from build123d import *

# Parameters (mm, degrees)
SKETCH1_W           = 25.4
SKETCH1_H           = 25.4
SKETCH1_W_2         = 20.32
SKETCH1_H_2         = 20.32
BOSS_EXTRUDE1_DEPTH = 139.7
SKETCH2_R           = 2.032
CUT_EXTRUDE1_DEPTH  = 143.557146436
SKETCH3_R           = 2.032
CUT_EXTRUDE2_DEPTH  = 143.557146436


with BuildPart() as part:
    # Sketch1 → Boss-Extrude1 (new body)
    with BuildSketch(Plane(origin=(0, 0, 0), x_dir=(0, 0, -1), z_dir=(1, 0, 0))):
        Rectangle(SKETCH1_W, SKETCH1_H)
        Rectangle(SKETCH1_W_2, SKETCH1_H_2, mode=Mode.SUBTRACT)
    extrude(amount=BOSS_EXTRUDE1_DEPTH)

    # Sketch2 → Cut-Extrude1 (cut, through all)
    with BuildSketch(Plane(origin=(0, 12.7, 0), x_dir=(1, 0, 0), z_dir=(0, 1, 0))):
        Circle(SKETCH2_R)
        with Locations(Location((12.7, 0, 0), (0, 0, 270))):
            Circle(SKETCH2_R)
        with Locations(Location((25.4, 0, 0), (0, 0, 270))):
            Circle(SKETCH2_R)
        with Locations(Location((38.1, 0, 0), (0, 0, 270))):
            Circle(SKETCH2_R)
        with Locations(Location((50.8, 0, 0), (0, 0, 270))):
            Circle(SKETCH2_R)
        with Locations(Location((63.5, 0, 0), (0, 0, 270))):
            Circle(SKETCH2_R)
        with Locations(Location((76.2, 0, 0), (0, 0, 270))):
            Circle(SKETCH2_R)
        with Locations(Location((88.9, 0, 0), (0, 0, 270))):
            Circle(SKETCH2_R)
        with Locations(Location((101.6, 0, 0), (0, 0, 270))):
            Circle(SKETCH2_R)
        with Locations(Location((114.3, 0, 0), (0, 0, 270))):
            Circle(SKETCH2_R)
        with Locations(Location((127, 0, 0), (0, 0, 270))):
            Circle(SKETCH2_R)
        with Locations((139.7, 0)):
            Circle(SKETCH2_R)
        with Locations((152.4, 0)):
            Circle(SKETCH2_R)
        with Locations((165.1, 0)):
            Circle(SKETCH2_R)
        with Locations((177.8, 0)):
            Circle(SKETCH2_R)
        with Locations((190.5, 0)):
            Circle(SKETCH2_R)
    extrude(amount=-CUT_EXTRUDE1_DEPTH, mode=Mode.SUBTRACT)

    # Sketch3 → Cut-Extrude2 (cut, through all)
    with BuildSketch(Plane(origin=(0, 0, -12.7), x_dir=(-1, 0, 0), z_dir=(0, 0, -1))):
        Circle(SKETCH3_R)
        with Locations((-12.7, 0)):
            Circle(SKETCH3_R)
        with Locations((-25.4, 0)):
            Circle(SKETCH3_R)
        with Locations((-38.1, 0)):
            Circle(SKETCH3_R)
        with Locations((-50.8, 0)):
            Circle(SKETCH3_R)
        with Locations((-63.5, 0)):
            Circle(SKETCH3_R)
        with Locations((-76.2, 0)):
            Circle(SKETCH3_R)
        with Locations((-88.9, 0)):
            Circle(SKETCH3_R)
        with Locations((-101.6, 0)):
            Circle(SKETCH3_R)
        with Locations((-114.3, 0)):
            Circle(SKETCH3_R)
        with Locations((-127, 0)):
            Circle(SKETCH3_R)
        with Locations((-139.7, 0)):
            Circle(SKETCH3_R)
        with Locations((-152.4, 0)):
            Circle(SKETCH3_R)
        with Locations((-165.1, 0)):
            Circle(SKETCH3_R)
        with Locations((-177.8, 0)):
            Circle(SKETCH3_R)
        with Locations((-190.5, 0)):
            Circle(SKETCH3_R)
        with Locations((-203.2, 0)):
            Circle(SKETCH3_R)
    extrude(amount=-CUT_EXTRUDE2_DEPTH, mode=Mode.SUBTRACT)


solid = part.part
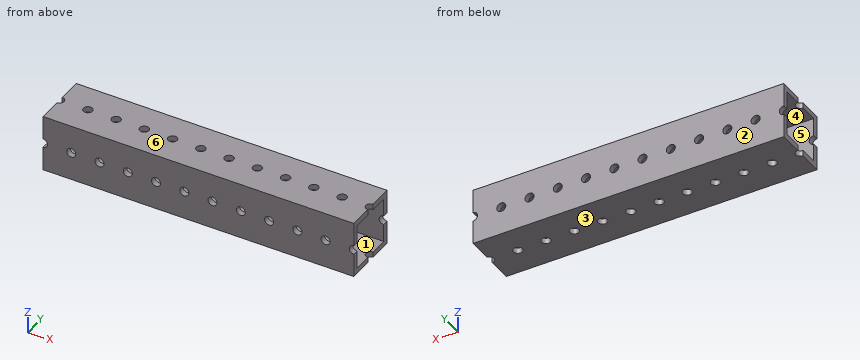
For this review, take the finished solid that the model builds, in its own axes (mm). Face numbers are marked on the shaded views. A direction names the side the tool comes from. Give positions to 0.01 mm unless a question says otherwise; leave off trailing zeros. Loops run counter-clockwise (first coordinate to the right, second up) from the corner with the lowest first, then second, coordinate; pieces in that order, holes last. Notation, with made-up numbers: M 24,-1 L 57,-1 A35 cw 57,33 Z; hole C 70.25,55.25 d10. An arc over 180 degrees is marked long. Put each result on its own line as item: value. Start each with the question number.
(1) The part is to be moulded in two halves that separate along Z. For the marked faces 1, 2, 3 and 4, say which applies: +Z half, -Z half, draft (parallel to the pull), parting line (faces both ways), or undercut.
(2) Add section B-B, the plane x = 114.3. Write out the cut boundary in (y, z), then the cut area to 3 significant figures.
(3) For pin 1 (6.5 mm diameter, centred on x = 88.9, z = 0, fed in from -Y), flat-tipped, find the tip position at first contact; note if it passes through.
(4) Machinability: for the marked faces 5 and 6, which of the approach directions +Z, -Z, +X, -X, +Y, -Y give a long, thin tool a straight path to every point of the face, cutting with its end or side? Answer none if there is none.
(5) Add section D-D, the plane y = 0. Give the number of separate pieces and of enclosed holes in the cut face, then the cut area to 3 significant figures.
(6) Add section A-A, the plane z = 4.25. Write out the cut boundary in (x, y).
(7) Wall thickness on L1, parallel to Z at x = 48.5, y = 2.75; L2, parallel to Y at x = 50.8, z = 10.9: over which ranges is each line inside the solid? List them lowest first.
Result:
1. face 1: undercut
1. face 2: draft
1. face 3: -Z half
1. face 4: undercut
2. outline: M -12.7,-12.7 L -2.03,-12.7 L -2.03,-10.16 L -10.16,-10.16 L -10.16,-2.03 L -12.7,-2.03 Z; M -12.7,2.03 L -10.16,2.03 L -10.16,10.16 L -2.03,10.16 L -2.03,12.7 L -12.7,12.7 Z; M 2.03,-12.7 L 12.7,-12.7 L 12.7,-2.03 L 10.16,-2.03 L 10.16,-10.16 L 2.03,-10.16 Z; M 2.03,10.16 L 10.16,10.16 L 10.16,2.03 L 12.7,2.03 L 12.7,12.7 L 2.03,12.7 Z
2. area: 191 mm^2
3. pin 1: stops at y = -12.7
4. face 5: +X, -X
4. face 6: +Z, +X, -X, +Y, -Y
5. separate pieces: 22
5. enclosed holes: 0
5. area: 483 mm^2
6. outline: M 0,-12.7 L 139.7,-12.7 L 139.7,-10.16 L 0,-10.16 Z; M 0,10.16 L 139.7,10.16 L 139.7,12.7 L 0,12.7 Z
7. L1: z = -12.7 to -10.16, 10.16 to 12.7
7. L2: y = -12.7 to -2.03, 2.03 to 12.7
